Study the drawing (mm; zero at the part's minimum x, y, z) and answer. Coordinates: 2 decimals unless noted, no trailing zeros. Loops run counter-clockwise (first coordinate to the right, second up) from the corner with the lowest first, then second, coordinate; pieces in that order, holes last. Notation, with made-up numbers: (54, -1.75) -> (80, -1.75) arc R18 ccw to (80, 31.25) -> close; hole circle Ø3 at (-15, 29). An arc over 180 degrees is marked (long way). Answer as a JSON object with one key per item and string values. Group by question number.
Q1. The part is cut by section A-A on z = 36. Write down the section's boundary in (x, y).
Q2. The part is cut by section B-B on y = 142.5. Write down the section's boundary in (x, z).
Q3. Straight lines are drawn through the part: line 1 along Z through (x, y) = (1.75, 162.5); line 2 along Y through (x, z) = (1.95, 36). For each, find the intervals that lie inside material, in ascending order. Write a range as [from, to].
Q4. This flat-tipped pin is pushed along its axis until it touches: P1, Ø3, axis at y = 162.5, z = 12, coming from the -X side. Where does it stop, or does it pass through?
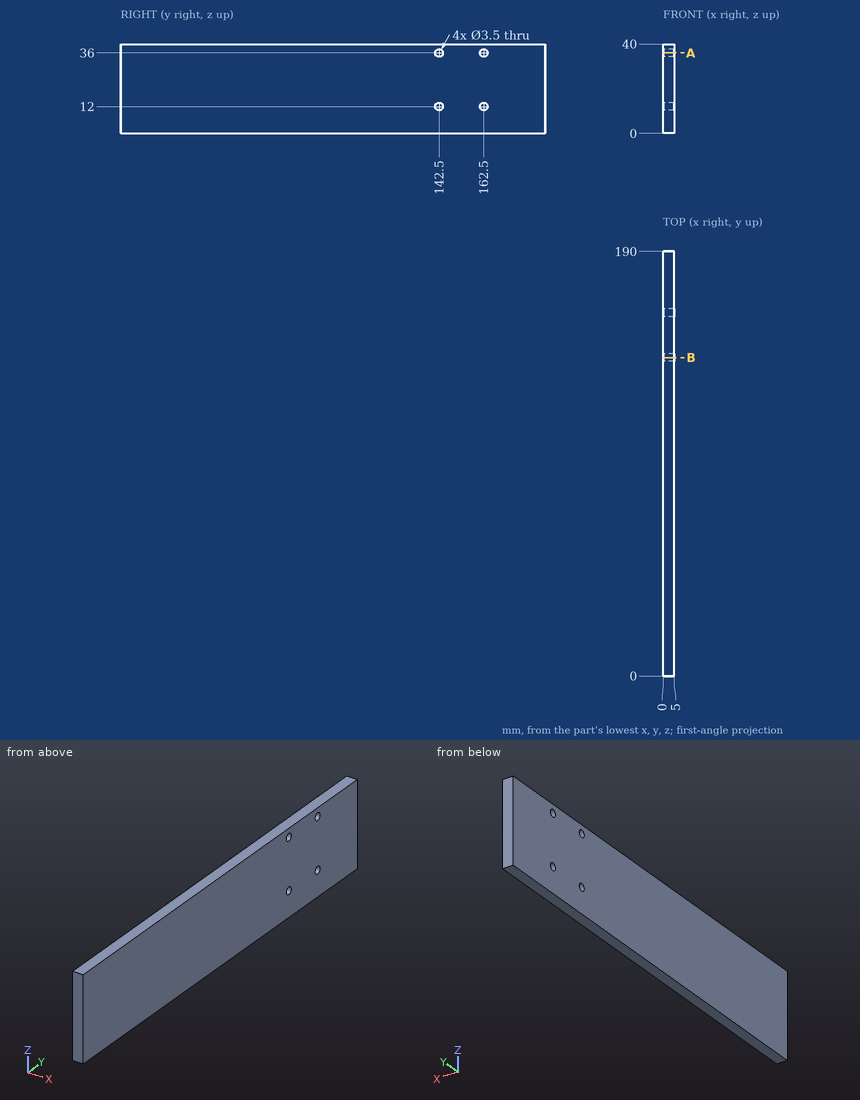
Final values:
{
 "1": {"outline": "(0, 0) -> (5, 0) -> (5, 140.75) -> (0, 140.75) -> close; (0, 144.25) -> (5, 144.25) -> (5, 160.75) -> (0, 160.75) -> close; (0, 164.25) -> (5, 164.25) -> (5, 190) -> (0, 190) -> close"},
 "2": {"outline": "(0, 0) -> (5, 0) -> (5, 10.25) -> (0, 10.25) -> close; (0, 13.75) -> (5, 13.75) -> (5, 34.25) -> (0, 34.25) -> close; (0, 37.75) -> (5, 37.75) -> (5, 40) -> (0, 40) -> close"},
 "3": {"line 1": "z = [0, 10.25], [13.75, 34.25], [37.75, 40]", "line 2": "y = [0, 140.75], [144.25, 160.75], [164.25, 190]"},
 "4": {"P1": "passes through"}
}
